Part model, mm, in its own coordinate system. A direction names the side the tool comes from. Coordinates: 2 decimals unless noted, no trailing zeros. Loops run counter-clockwise (first coordinate to the right, second up) from the corner with the lowest first, then second, coordinate; pieces in that order, holes last. Notation, with made-up numbers: (84.25, 50) - (108.25, 50) arc R25 ccw to (108.25, 68) - close; hole circle Ø5 at (9, 59). An arc over 180 degrees is marked (long way). Use a Markdown table: item, result. Add a question column.
1) Band-saw the part on C-C (x = -65). Give the cut face in (y, z) (3 decimals).
2) Band-saw the part on A-A (y = -0.6). Give the cut face in (x, z) (1 decimal).
3) Band-saw the part on B-B (z = 71.5). Give the cut face in (x, y) (3 decimals), plus the area to 3 significant figures.
4) Pull direction Z, two halves, no side cores. Call faces 1 (the face through (-89.55, -1.57, 134.14)), 2 (the face through (-30.409, -1.565, 43.664)), 3 (the face through (-29.428, -1.565, 129.989)): +Z half, -Z half, draft (parallel to the pull), parting line (faces both ways), or undercut.
5) Probe probe 1 along Z at (x, y) = (-102, -1.35); probe 2 along Z at (x, y) = (-34.5, -1.4); probe 3 along X at (y, z) = (-2.1, 157). List the from-to ranges inside material, lowest first. Write a range as [from, to].
6) Tool access for faces 4 (the face through (-29.6, -1.6, 135.3)), 5 (the face through (-28.615, -1.565, 46.644)), 6 (the face through (-90.387, -1.565, 42.458)), 7 (the face through (-93.3, -1.57, 133.97)): list every direction of +Z, -Z, +X, -X, +Y, -Y with a clear straight run to the whole face (end or side of a thin tool).
from build123d import *

# Parameters (mm, degrees)
F1_DEPTH = 3.175


with BuildPart() as f1:
    # F0 (on Front) → F1 (new body)
    with BuildSketch(Plane.XZ):
        Polygon((-119.95591, 177.8), (-123.825, 177.8), (-61.9125, 88.9), (-59.977955, 91.677808), align=None)
        Polygon((-59.977955, 86.122192), (0, 0), (0, 5.555616), (-58.04341, 88.9), align=None)
        Polygon((-123.825, 0), (-119.95591, 0), (-59.977955, 86.122192), (-58.04341, 88.9), (0, 172.244384), (0, 177.8), (-59.977955, 91.677808), (-61.9125, 88.9), align=None)
    extrude(amount=F1_DEPTH)


solid = f1.part
Answer block:
| question | item | result |
|---|---|---|
| 1 | outline | (-3.175, 78.911) - (0, 78.911) - (0, 84.467) - (-3.175, 84.467) - close; (-3.175, 93.333) - (0, 93.333) - (0, 98.889) - (-3.175, 98.889) - close |
| 2 | outline | (-123.8, 0) - (-120, 0) - (-60, 86.1) - (0, 0) - (0, 5.6) - (-58, 88.9) - (0, 172.2) - (0, 177.8) - (-60, 91.7) - (-120, 177.8) - (-123.8, 177.8) - (-61.9, 88.9) - close |
| 3 | outline | (-74.03, -3.175) - (-70.161, -3.175) - (-70.161, 0) - (-74.03, 0) - close; (-49.795, -3.175) - (-45.926, -3.175) - (-45.926, 0) - (-49.795, 0) - close |
| 3 | area | 24.6 mm2 |
| 4 | face 1 | +Z half |
| 4 | face 2 | -Z half |
| 4 | face 3 | undercut |
| 5 | probe 1 | [25.78, 31.34], [146.46, 152.02] |
| 5 | probe 2 | [49.54, 55.09], [122.71, 128.26] |
| 5 | probe 3 | [-109.34, -105.47], [-14.49, -10.62] |
| 6 | face 4 | +Z, +Y, -Y |
| 6 | face 5 | +X, +Y, -Y |
| 6 | face 6 | -Z, +Y, -Y |
| 6 | face 7 | -X, +Y, -Y |
